```python
from build123d import *

# Parameters (mm, degrees)
F1_DEPTH = 25.4
F2_D     = 12.7
F3_SIZE  = 50.8


with BuildPart() as f1:
    # F0 (on Top) → F1 (new body)
    with BuildSketch(Plane.XY):
        Polygon((48.011348, -83.158093), (48.011348, 83.158093), (-96.022695, 0), align=None)
    extrude(amount=F1_DEPTH)

    # F2 (through all)
    with Locations(Plane(origin=(0, 0, 0), x_dir=(1, 0, 0), z_dir=(0, 0, -1))):
        with Locations((0, 0)):
            Hole(F2_D / 2)

    # F3
    f3_edges = [f1.edges().sort_by_distance(p)[0] for p in [
        (48.011348, -83.158093, 12.7),
        (48.011348, 83.158093, 12.7),
        (-96.022695, 0, 12.7),
    ]]
    chamfer(f3_edges, length=F3_SIZE)


solid = f1.part
```
Model file for the job. Use its own axes, mm. Coordinates: 2 decimals unless noted, no trailing zeros. Order: outer loops, then holes, each group sorted by start corner. A loop starts at its lowest first (then second) coordinate and runs counter-clockwise, first axis right, second up. Notation, with made-up numbers: (69.25, 35) -> (124.25, 35) arc R25 ccw to (124.25, 51) -> close; hole circle Ø11 at (58.25, 15). An arc over 180 degrees is marked (long way). Answer as a JSON object with one key per item and string values. Group by question number.
1) Cut at D-D, the plane x = 36.5. Write the cut outline in (y, z), then the cut area to 3 significant figures.
2) Flat gauge pins, fed straight in: pin 1 (2 mm diameter, centred on x = 16.5, z = 8.5, fed in from +Y); pin 2 (14.5 mm diameter, centred on x = 0, y = 0, fed in from -Z); pin 3 (8 mm diameter, centred on x = 17, z = 13.5, fed in from +Y); pin 4 (3 mm diameter, centred on y = 33, z = 12.5, fed in from -X). Where does each tip first touch, or does it go through?
3) Cut at A-A, the plane y = 0. Write the cut outline in (x, z).
4) Cut at C-C, the plane x = 0. Write the cut outline in (y, z), then the cut area to 3 significant figures.
5) Cut at B-B, the plane z = 15.75. Write the cut outline in (x, y), then the cut area to 3 significant figures.
6) Drill centre lines: L1, parallel to Y at x = 0, z = 11.25; L2, parallel to Y at x = 29, z = 12.75; L3, parallel to X at y = -50.5, z = 11.5. Where is each one in solid material? Low to high.
Check values:
{
 "1": {"outline": "(-39, 0) -> (39, 0) -> (39, 25.4) -> (-39, 25.4) -> close", "area": "1,980 mm²"},
 "2": {"pin 1": "stops at y = 51.13", "pin 2": "stops at z = 0", "pin 3": "stops at y = 52.57", "pin 4": "stops at x = -41.46"},
 "3": {"outline": "(-52.03, 0) -> (-6.35, 0) -> (-6.35, 25.4) -> (-52.03, 25.4) -> close; (6.35, 0) -> (48.01, 0) -> (48.01, 25.4) -> (6.35, 25.4) -> close"},
 "4": {"outline": "(-55.44, 0) -> (-6.35, 0) -> (-6.35, 25.4) -> (-55.44, 25.4) -> close; (6.35, 0) -> (55.44, 0) -> (55.44, 25.4) -> (6.35, 25.4) -> close", "area": "2,490 mm²"},
 "5": {"outline": "(-52.03, -25.4) -> (4.02, -57.76) -> (48.01, -32.36) -> (48.01, 32.36) -> (4.02, 57.76) -> (-52.03, 25.4) -> close; hole circle Ø12.7 at (0, 0)", "area": "8,500 mm²"},
 "6": {"L1": "y = -55.44 to -6.35, 6.35 to 55.44", "L2": "y = -43.33 to 43.33", "L3": "x = -8.55 to 16.59"}
}
